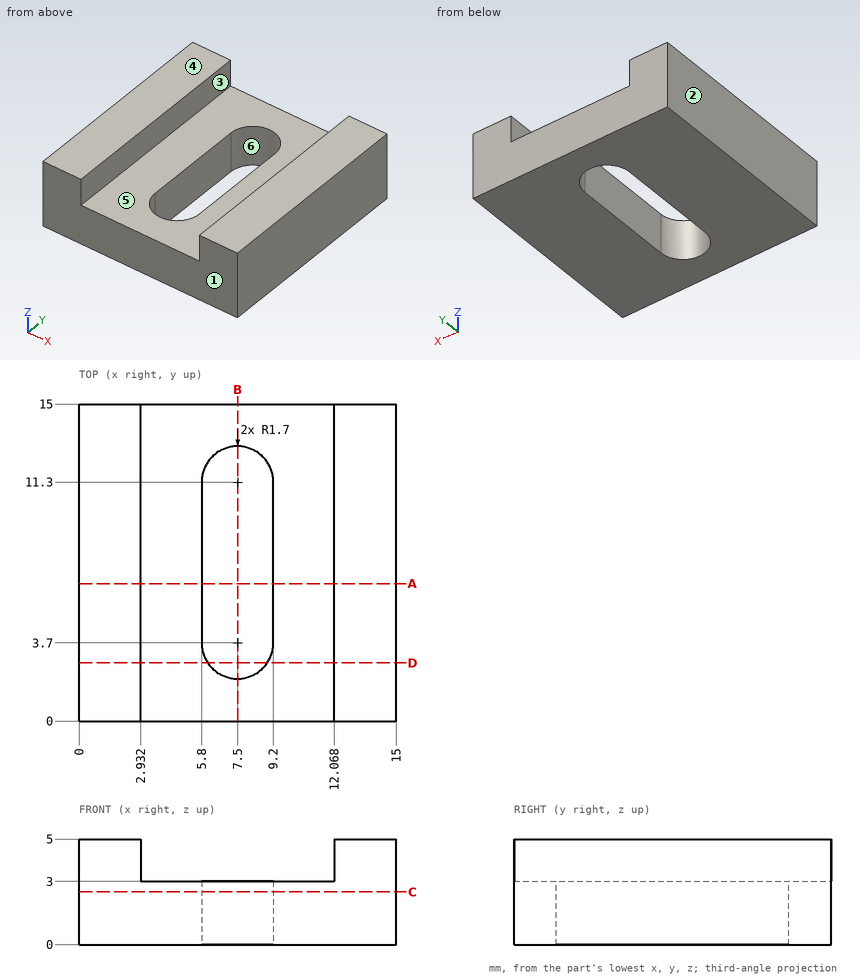
The drawing under review shows one solid part. Ordinate dimensions are in mm from its lowest x, y, z. A direction names the side the tool comes from. Give positions to 0.01 mm unless a question says otherwise; leave off trailing zeros. Write each loop counter-clockwise with the first axis right and the second up, starting at its lowest first coordinate (ties: lowest second). Pieces come first, ordered by that corner, then holes. Notation, with made-up numbers: (-25, -24.75) - (19, -24.75) arc R23 cw to (19, -7.75) - close; hole circle Ø8 at (63, 43). An arc over 180 degrees is marked (long way). Answer in a Markdown table with one row per item. Add a question column.
1. Tool access review of the marked faces 4, 5 and 6: name each direction out of +Z, -Z, +X, -X, +Y, -Y from which nothing blocks a thin tool from reaching the whole face with its end or side.
2. We need section A-A on y = 6.5. Write out the cut boundary in (x, z), then the cut area to 3 significant figures.
3. Wall thickness on line 1 along X through (y, z) = (13, 3.1); line 2 along X through (y, z) = (9.5, 1.8); line 3 along Y through (x, z) = (6.5, 0.5) (1 decimal): over which ranges is each line inside the solid? List them lowest first. Write a range as [from, to].
4. We need section C-C on z = 2.5. Write out the cut boundary in (x, y), then the cut area to 3 significant figures.
5. Insertion check: P1, Ø1.6, axis at y = 5.5, z = 3.5, coming from the -X side; P2, Ø2, axis at x = 5, y = 13.5, coming from the +Z side. Each pin has a flat end and moves straight along its axis. Give the tip position at first contact, or say it passes through.
6. We need section B-B on x = 7.5. Write out the cut boundary in (y, z).
7. Draft analysis for pull direction X (two halves, no side actions). For the marked faces 1, 2 and 3, state which applies: +X half, -X half, draft (parallel to the pull), parting line (faces both ways), or undercut.
8. We need section D-D on y = 2.75. Write out the cut boundary in (x, z).
Ans:
| question | item | result |
|---|---|---|
| 1 | face 4 | +Z, +X, -X, +Y, -Y |
| 1 | face 5 | +Z, +Y, -Y |
| 1 | face 6 | +Z, -Z |
| 2 | outline | (0, 0) - (5.8, 0) - (5.8, 3) - (2.93, 3) - (2.93, 5) - (0, 5) - close; (9.2, 0) - (15, 0) - (15, 5) - (12.07, 5) - (12.07, 3) - (9.2, 3) - close |
| 2 | area | 46.5 mm^2 |
| 3 | line 1 | x = [0, 2.93], [12.07, 15] |
| 3 | line 2 | x = [0, 5.8], [9.2, 15] |
| 3 | line 3 | y = [0, 2.3], [12.7, 15] |
| 4 | outline | (0, 0) - (15, 0) - (15, 15) - (0, 15) - close; hole (5.8, 3.7) arc R1.7 ccw to (9.2, 3.7) - (9.2, 11.3) arc R1.7 ccw to (5.8, 11.3) - close |
| 4 | area | 190 mm^2 |
| 5 | P1 | stops at x = 0 |
| 5 | P2 | stops at z = 3 |
| 6 | outline | (0, 0) - (2, 0) - (2, 3) - (0, 3) - close; (13, 0) - (15, 0) - (15, 3) - (13, 3) - close |
| 7 | face 1 | draft |
| 7 | face 2 | -X half |
| 7 | face 3 | undercut |
| 8 | outline | (0, 0) - (6.09, 0) - (6.09, 3) - (2.93, 3) - (2.93, 5) - (0, 5) - close; (8.91, 0) - (15, 0) - (15, 5) - (12.07, 5) - (12.07, 3) - (8.91, 3) - close |
